Geometry check sheet. Reference: the model listing, model coordinates, mm. A direction names the side the tool comes from. Round coordinates to 2 decimals unless told otherwise and drop trailing zeros. Write each loop counter-clockwise with the first axis right and the second up, starting at its lowest first coordinate (ties: lowest second). Pieces come first, ordered by that corner, then holes. Notation, with made-up numbers: (23, 30) - (37, 30) arc R10 cw to (37, 48) - close; hole circle Ø5 at (63, 80.5). An arc over 180 degrees is marked (long way). Return JSON: item names as keys, results as strings.
```python
from build123d import *

# Parameters (mm, degrees)
SKETCH1_R           = 12.5
SKETCH1_R_2         = 8
SKETCH1_R_3         = 13
BOSS_EXTRUDE1_DEPTH = 5
CUT_EXTRUDE1_DEPTH  = 3


with BuildPart() as part:
    # Sketch1 → Boss-Extrude1 (new, symmetric)
    # profile 1 of 3: a face of its own
    with BuildSketch(Plane.XY):
        with BuildLine():
            Line((-12.463466587, 130.955210764), (-22.23722085, 3.428703671))
            ThreePointArc((-22.23722085, 3.428703671), (-5.852e-06, 22.5), (22.237219067, 3.428715237))
            Line((22.237219067, 3.428715237), (12.463432081, 130.955214005))
            ThreePointArc((12.463432081, 130.955214005), (12.490841831, 130.477956524), (12.499982871, 130))
            ThreePointArc((12.499982871, 130), (-0.477972029, 117.509140978), (-12.463466587, 130.955210764))
        make_face()
    # profile 2 of 3: a face of its own
    with BuildSketch(Plane.XY):
        with Locations((-1.7129e-05, 130)):
            Circle(SKETCH1_R)
        with Locations((-1.7129e-05, 130)):
            Circle(SKETCH1_R_2, mode=Mode.SUBTRACT)
    # profile 3 of 3: a face of its own
    with BuildSketch(Plane.XY):
        with BuildLine():
            Line((-22.23722085, 3.428703671), (-22.5, 0))
            ThreePointArc((-22.5, 0), (0, -22.5), (22.5, 0))
            Line((22.5, 0), (22.237219067, 3.428715237))
            ThreePointArc((22.237219067, 3.428715237), (-5.852e-06, 22.5), (-22.23722085, 3.428703671))
        make_face()
        Circle(SKETCH1_R_3, mode=Mode.SUBTRACT)
    extrude(amount=BOSS_EXTRUDE1_DEPTH, both=True)

    # Sketch2 → Cut-Extrude1 (cut)
    with BuildSketch(Plane.XY.offset(5)):
        with BuildLine():
            Line((17.041069078, 5.796720166), (8.289478443, 119.985796928))
            ThreePointArc((8.289478443, 119.985796928), (-1.5438e-05, 117), (-8.289510096, 119.985794772))
            Line((-8.289510096, 119.985794772), (-17.041071164, 5.796714033))
            ThreePointArc((-17.041071164, 5.796714033), (-3.239e-06, 18), (17.041069078, 5.796720166))
        make_face()
    cut_extrude1 = extrude(amount=-CUT_EXTRUDE1_DEPTH, mode=Mode.SUBTRACT)

    # Mirror1: Cut-Extrude1 across plane
    add(cut_extrude1.mirror(Plane.XY), mode=Mode.SUBTRACT)


solid = part.part
```
(1) Access from +Z, -Z, +X, -X, +Y, -Y to the whole of each face (thin tool, end or side, straight path). Record for faces 1 (the face through (12.727, 62.092, -3.521)), 2 (the face through (-12.604, 63.691, 3.521)), 3 (the face through (0.261, 142.497, 0.07)).
Response values:
{"face 1": "-Z", "face 2": "+Z", "face 3": "+Z, -Z, +Y"}
(2) Section check B-B, the plane x = 11. Enter the section's corners in (y, z), plus the area to 3 significant figures.
Response values:
{"outline": "(-19.63, -5) - (-6.93, -5) - (-6.93, 5) - (-19.63, 5) - close; (6.93, -5) - (14.25, -5) - (14.25, -2) - (84.62, -2) - (84.62, -5) - (135.94, -5) - (135.94, 5) - (84.62, 5) - (84.62, 2) - (14.25, 2) - (14.25, 5) - (6.93, 5) - close", "area": "995 mm^2"}
(3) Section check A-A, the plane x = 0. Enter the section's corners in (y, z).
Response values:
{"outline": "(-22.5, -5) - (-13, -5) - (-13, 5) - (-22.5, 5) - close; (13, -5) - (18, -5) - (18, -2) - (117, -2) - (117, -5) - (122, -5) - (122, 5) - (117, 5) - (117, 2) - (18, 2) - (18, 5) - (13, 5) - close; (138, -5) - (142.5, -5) - (142.5, 5) - (138, 5) - close"}
(4) Material ranges on line 1 along Y through (x, z) = (0, -0.75); line 2 along Y through (x, z) = (-5.5, 2.5); line 3 along Z through (x, y) = (0.5, 34), recorded low to high. Write a range as [from, to].
Response values:
{"line 1": "y = [-22.5, -13], [13, 122], [138, 142.5]", "line 2": "y = [-21.82, -11.78], [11.78, 17.14], [118.22, 124.19], [135.81, 141.22]", "line 3": "z = [-2, 2]"}
(5) Section check C-C, the plane y = 105. Enter the section's corners in (x, z), plus the area to 3 significant figures.
Response values:
{"outline": "(-14.45, -5) - (-9.44, -5) - (-9.44, -2) - (9.44, -2) - (9.44, -5) - (14.45, -5) - (14.45, 5) - (9.44, 5) - (9.44, 2) - (-9.44, 2) - (-9.44, 5) - (-14.45, 5) - close", "area": "176 mm^2"}
(6) Gauge pin test, flat ends, axial feed: pin 1 (1.5 mm diameter, centred on x = 5, y = 32, fed in from +Z); pin 2 (3 mm diameter, centred on x = 0.5, z = 0.5, fed in from -Y); pin 3 (6 mm diameter, centred on y = 17.5, z = -3, fed in from -X). Record the tip position at first contact, or that the pin passes through.
Response values:
{"pin 1": "stops at z = 2", "pin 2": "stops at y = -22.5", "pin 3": "stops at x = -21.39"}
